The listing builds one solid part. Answer for the finished solid, in the listing's coordinates (mm). Face numbers are marked on the shaded views. A direction names the side the tool comes from. Coordinates: 2 decimals unless noted, no trailing zeros. Loops run counter-clockwise (first coordinate to the right, second up) from the corner with the lowest first, then second, coordinate; pieces in that order, holes last. Notation, with made-up numbers: (46.25, -26) - (56.25, -26) arc R29 ccw to (56.25, -2) - close; hole circle Ø5 at (64.25, 77). An arc over 180 degrees is marked (long way). Put each result on its own line as item: value.
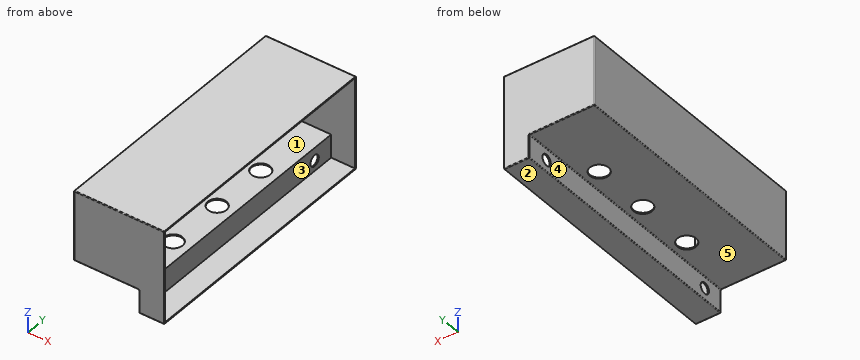
```python
from build123d import *

# Parameters (mm, degrees)
EXTRUDE_1_DEPTH              = 165
SHELL_1_T                    = -0.8
SKETCH_2_R                   = 6
CUT_EXTRUDE_4_DEPTH          = 1
FILLET_1_R                   = 0.5
HOLE_WIZARD_9_32_0_28125_1_D = 7.14375


with BuildPart() as part:
    # 草图1 → 凸台-拉伸1 (new body)
    with BuildSketch(Plane(origin=(0, 0, 0), x_dir=(1, 0, 0), z_dir=(0, 1, 0))):
        Polygon((3, 5), (3, -55), (-55, -55), (-55, -10), (-13.1, -10), (-13.1, 5), align=None)
    extrude(amount=EXTRUDE_1_DEPTH)

    # 抽壳1
    shell_1_openings = [part.faces().sort_by_distance(p)[0] for p in [
        (3, 82.5, 25),
    ]]
    offset(amount=SHELL_1_T, openings=shell_1_openings, kind=Kind.INTERSECTION)

    # 草图2 → 切除-拉伸4 (cut)
    with BuildSketch(Plane(origin=(0, 0, 10), x_dir=(-1, 0, 0), z_dir=(0, 0, -1))):
        with Locations((23, 42.75)):
            Circle(SKETCH_2_R)
        with Locations((23, 118)):
            Circle(SKETCH_2_R)
        with Locations((23, 80.55)):
            Circle(SKETCH_2_R)
    extrude(amount=-CUT_EXTRUDE_4_DEPTH, mode=Mode.SUBTRACT)

    # 圆角1
    fillet_1_edges = [part.edges().sort_by_distance(p)[0] for p in [
        (-55, 82.5, 55),
        (-55, 82.5, 10),
        (-13.1, 82.5, 10),
        (-13.1, 82.5, -5),
        (-34.05, 165, 10),
        (-55, 165, 32.5),
        (-26, 165, 55),
        (-5.05, 165, -5),
        (-26, 0, 55),
        (-55, 0, 32.5),
        (-34.05, 0, 10),
        (-13.1, 0, 2.5),
        (-5.05, 0, -5),
        (-13.1, 165, 2.5),
    ]]
    fillet(fillet_1_edges, radius=FILLET_1_R)

    # 9/32 (0.28125) 直径孔1 (through all)
    with Locations(Plane.ZY.offset(13.1)):
        with Locations((2.5, 150), (2.5, 14)):
            Hole(HOLE_WIZARD_9_32_0_28125_1_D / 2)


solid = part.part
```
1) The part is cut by section C-C (z = 29). Give the vertices of the cut face in (x, y).
Found:
outline: (-55, 0.5) arc R0.5 ccw to (-54.5, 0) - (3, 0) - (3, 0.8) - (-54.2, 0.8) - (-54.2, 164.2) - (3, 164.2) - (3, 165) - (-54.5, 165) arc R0.5 ccw to (-55, 164.5) - close
2) The part is cut by section B-B (y = 80.55). Give the vertices of the cut face in (x, z).
Found:
outline: (-55, 10.5) arc R0.5 ccw to (-54.5, 10) - (-29, 10) - (-29, 10.8) - (-54.2, 10.8) - (-54.2, 54.2) - (3, 54.2) - (3, 55) - (-54.5, 55) arc R0.5 ccw to (-55, 54.5) - close; (-17, 10) - (-13.6, 10) arc R0.5 cw to (-13.1, 9.5) - (-13.1, -4.5) arc R0.5 ccw to (-12.6, -5) - (3, -5) - (3, -4.2) - (-12.3, -4.2) - (-12.3, 10.8) - (-17, 10.8) - close
3) Straight lines are drawn through the part: L1, parallel to Y at x = -12, z = 2; L2, parallel to Z at x = -22.5, y = 11; L3, parallel to Z at x = -12, y = 14. For each, find the intervals that lie inside material, in ascending order. Write a range as [from, to].
Found:
L1: y = [0, 0.8], [164.2, 165]
L2: z = [10, 10.8], [54.2, 55]
L3: z = [-5, -4.2], [54.2, 55]
4) For the marked faces 1 and 2, determine the directions among +Z, -Z, +X, -X, +Y, -Y from which every point of the face is accessible in a straight line to the end or side of a thin tool.
Found:
face 1: +X
face 2: -Z, +X, -X, +Y, -Y
5) For a pull along Z with two mould halves and no side action, classify the marked faces 3, 4 and 5 as pulls with the +Z half, pulls with the -Z half, needs draft (parallel to the pull), parting line crosses it, or undercut.
Found:
face 3: undercut
face 4: needs draft
face 5: pulls with the -Z half
6) Each of these flat-tipped pins is pushed along its axis until it touches: pin 1 (4.5 mm diameter, centred on y = 14, z = 2.5, fed in from -X); pin 2 (4.5 mm diameter, centred on y = 73.5, z = 6.5, fed in from +X); pin 3 (7 mm diameter, centred on y = 80.5, z = 2, fed in from -X); pin 4 (12.5 mm diameter, centred on x = -42.5, y = 116.5, fed in from -Z). Where does it stop, or does it pass through?
Found:
pin 1: passes through
pin 2: stops at x = -12.3
pin 3: stops at x = -13.1
pin 4: stops at z = 10
7) The part is cut by section D-D (x = -23). Give the vertices of the cut face in (y, z).
Found:
outline: (0, 10.5) arc R0.5 ccw to (0.5, 10) - (36.75, 10) - (36.75, 10.8) - (0.8, 10.8) - (0.8, 54.2) - (164.2, 54.2) - (164.2, 10.8) - (124, 10.8) - (124, 10) - (164.5, 10) arc R0.5 ccw to (165, 10.5) - (165, 54.5) arc R0.5 ccw to (164.5, 55) - (0.5, 55) arc R0.5 ccw to (0, 54.5) - close; (48.75, 10) - (74.55, 10) - (74.55, 10.8) - (48.75, 10.8) - close; (86.55, 10) - (112, 10) - (112, 10.8) - (86.55, 10.8) - close
8) The part is cut by section A-A (x = -49). Give the vertices of the cut face in (y, z), and give its area (3 significant figures).
Found:
outline: (0, 10.5) arc R0.5 ccw to (0.5, 10) - (164.5, 10) arc R0.5 ccw to (165, 10.5) - (165, 54.5) arc R0.5 ccw to (164.5, 55) - (0.5, 55) arc R0.5 ccw to (0, 54.5) - close; hole (0.8, 10.8) - (164.2, 10.8) - (164.2, 54.2) - (0.8, 54.2) - close
area: 333 mm^2
